Model file for the job. Use its own axes, mm. A direction names the side the tool comes from. Coordinates: 2 decimals unless noted, no trailing zeros. Write each loop counter-clockwise with the first axis right and the second up, starting at its lowest first coordinate (ties: lowest second). Pieces come first, ordered by that corner, then holes. Notation, with made-up numbers: (3.25, 58.25) - (58.25, 58.25) arc R13 ccw to (58.25, 70.25) - close; hole circle Ø8 at (-22, 52). An arc over 180 degrees is marked (long way). Put each result on its own line as item: value. Start each with the question number.
1. Pull direction Y, two halves, no side cores. Call faces 1 (the face through (10.19, 15, 99)), 2 (the face through (18.717, -18.647, 98.6)), 3 (the face through (-17, -2.966, 99)), 4 (the face through (5.385, 17, 99)): released by +Y, released by -Y, zero draft, split by the parting line, or undercut.
2. Which spindle directions (+Z, -Z, +X, -X, +Y, -Y) get a long thin tool onto all of the face, cutting with end or side? Do faces 5 (the face through (-11, -20, 99)), 6 (the face through (18.2, -8, 99)), 7 (the face through (17, 2.966, 99)). Say none if no direction does.
3. Saw through at A-A, the plane y = -8. Write the cut outline in (x, z), plus the area to 3 significant figures.
4. Saw through at B-B, the plane z = 111.5. Give the number of separate pieces and of enclosed holes in the cut face, plus the area to 3 significant figures.
5. Drill centre lines: L1, parallel to Y at x = 16, z = 160; L2, parallel to Y at x = -14, z = 22. Where is each one in solid material? Low to high. Write a range as from..to.
6. Drop flat-ended pins along their axis: P1, Ø2, axis at x = -3, y = 8, coming from the -Z side; P2, Ø2, axis at x = 17.5, z = 91, coming from the -Y side; P3, Ø0.8, axis at x = -19.5, z = 74, coming from the +Y side; P4, Ø1, axis at y = 1.5, z = 123.5, coming from the +X side. Give the stop position or say it passes through.
```python
from build123d import *

# Parameters (mm, degrees)
BOSS_EXTRUDE1_DEPTH  = 200
MIRROR3_COPY_1_DEPTH = 200
MIRROR3_COPY_2_DEPTH = 200


with BuildPart() as part:
    # Sketch1 → Boss-Extrude1 (new body)
    with BuildSketch(Plane.XY):
        with BuildLine():
            Line((3.4, 0), (5.5, 0))
            Line((5.5, 0), (5.5, 4))
            Line((5.5, 4), (11.69, 10.19))
            Line((11.69, 10.19), (18.2, 10.19))
            Line((18.2, 10.19), (18.2, 5.265595036))
            Line((18.2, 5.265595036), (15.5, 5.265595036))
            Line((15.5, 5.265595036), (15.5, 2.965595036))
            Line((15.5, 2.965595036), (19, 2.965595036))
            Line((19, 2.965595036), (19, 3.965595036))
            Line((19, 3.965595036), (20, 3.965595036))
            Line((20, 3.965595036), (20, 15.5))
            ThreePointArc((20, 15.5), (18.681980515, 18.681980515), (15.5, 20))
            Line((15.5, 20), (6.385304712, 20))
            Line((6.385304712, 20), (6.385304712, 19))
            Line((6.385304712, 19), (5.385304712, 19))
            Line((5.385304712, 19), (5.385304712, 15.5))
            Line((5.385304712, 15.5), (7.685304712, 15.5))
            Line((7.685304712, 15.5), (7.685304712, 18.2))
            Line((7.685304712, 18.2), (10.19, 18.2))
            Line((10.19, 18.2), (10.19, 11.69))
            Line((10.19, 11.69), (4, 5.5))
            Line((4, 5.5), (0, 5.5))
            Line((0, 5.5), (0, 3.4))
            ThreePointArc((0, 3.4), (2.404163056, 2.404163056), (3.4, 0))
        make_face()
        with BuildLine():
            Line((18.5, 11.69), (18.5, 15.5))
            ThreePointArc((18.5, 15.5), (17.621320344, 17.621320344), (15.5, 18.5))
            Line((15.5, 18.5), (11.69, 18.5))
            Line((11.69, 18.5), (11.69, 11.69))
            Line((11.69, 11.69), (18.5, 11.69))
        make_face(mode=Mode.SUBTRACT)
    boss_extrude1 = extrude(amount=BOSS_EXTRUDE1_DEPTH)

    # Mirror1: Boss-Extrude1 across plane
    add(boss_extrude1.mirror(Plane.ZX))

    # Mirror2: Boss-Extrude1 across plane
    add(boss_extrude1.mirror(Plane(origin=(0, 0, 0), x_dir=(0, 0, 1), z_dir=(1, 0, 0))))

    # Mirror3 copy 1 sketch → Mirror3 copy 1 (add)
    with BuildSketch(Plane(origin=(0, 0, 0), x_dir=(-1, 0, 0), z_dir=(0, 0, 1))):
        with BuildLine():
            Line((3.4, 0), (5.5, 0))
            Line((5.5, 0), (5.5, 4))
            Line((5.5, 4), (11.69, 10.19))
            Line((11.69, 10.19), (18.2, 10.19))
            Line((18.2, 10.19), (18.2, 5.265595036))
            Line((18.2, 5.265595036), (15.5, 5.265595036))
            Line((15.5, 5.265595036), (15.5, 2.965595036))
            Line((15.5, 2.965595036), (19, 2.965595036))
            Line((19, 2.965595036), (19, 3.965595036))
            Line((19, 3.965595036), (20, 3.965595036))
            Line((20, 3.965595036), (20, 15.5))
            ThreePointArc((20, 15.5), (18.681980515, 18.681980515), (15.5, 20))
            Line((15.5, 20), (6.385304712, 20))
            Line((6.385304712, 20), (6.385304712, 19))
            Line((6.385304712, 19), (5.385304712, 19))
            Line((5.385304712, 19), (5.385304712, 15.5))
            Line((5.385304712, 15.5), (7.685304712, 15.5))
            Line((7.685304712, 15.5), (7.685304712, 18.2))
            Line((7.685304712, 18.2), (10.19, 18.2))
            Line((10.19, 18.2), (10.19, 11.69))
            Line((10.19, 11.69), (4, 5.5))
            Line((4, 5.5), (0, 5.5))
            Line((0, 5.5), (0, 3.4))
            ThreePointArc((0, 3.4), (2.404163056, 2.404163056), (3.4, 0))
        make_face()
        with BuildLine():
            Line((18.5, 11.69), (18.5, 15.5))
            ThreePointArc((18.5, 15.5), (17.621320344, 17.621320344), (15.5, 18.5))
            Line((15.5, 18.5), (11.69, 18.5))
            Line((11.69, 18.5), (11.69, 11.69))
            Line((11.69, 11.69), (18.5, 11.69))
        make_face(mode=Mode.SUBTRACT)
    extrude(amount=MIRROR3_COPY_1_DEPTH)

    # Mirror3 copy 2 sketch → Mirror3 copy 2 (add)
    with BuildSketch(Plane.XY):
        with BuildLine():
            Line((3.4, 0), (5.5, 0))
            Line((5.5, 0), (5.5, -4))
            Line((5.5, -4), (11.69, -10.19))
            Line((11.69, -10.19), (18.2, -10.19))
            Line((18.2, -10.19), (18.2, -5.265595036))
            Line((18.2, -5.265595036), (15.5, -5.265595036))
            Line((15.5, -5.265595036), (15.5, -2.965595036))
            Line((15.5, -2.965595036), (19, -2.965595036))
            Line((19, -2.965595036), (19, -3.965595036))
            Line((19, -3.965595036), (20, -3.965595036))
            Line((20, -3.965595036), (20, -15.5))
            ThreePointArc((20, -15.5), (18.681980515, -18.681980515), (15.5, -20))
            Line((15.5, -20), (6.385304712, -20))
            Line((6.385304712, -20), (6.385304712, -19))
            Line((6.385304712, -19), (5.385304712, -19))
            Line((5.385304712, -19), (5.385304712, -15.5))
            Line((5.385304712, -15.5), (7.685304712, -15.5))
            Line((7.685304712, -15.5), (7.685304712, -18.2))
            Line((7.685304712, -18.2), (10.19, -18.2))
            Line((10.19, -18.2), (10.19, -11.69))
            Line((10.19, -11.69), (4, -5.5))
            Line((4, -5.5), (0, -5.5))
            Line((0, -5.5), (0, -3.4))
            ThreePointArc((0, -3.4), (2.404163056, -2.404163056), (3.4, 0))
        make_face()
        with BuildLine():
            Line((18.5, -11.69), (18.5, -15.5))
            ThreePointArc((18.5, -15.5), (17.621320344, -17.621320344), (15.5, -18.5))
            Line((15.5, -18.5), (11.69, -18.5))
            Line((11.69, -18.5), (11.69, -11.69))
            Line((11.69, -11.69), (18.5, -11.69))
        make_face(mode=Mode.SUBTRACT)
    extrude(amount=MIRROR3_COPY_2_DEPTH)


solid = part.part
```
Final values:
1. face 1: undercut
1. face 2: released by -Y
1. face 3: undercut
1. face 4: zero draft
2. face 5: +Z, -Z, +X, -X, -Y
2. face 6: +Z, -Z
2. face 7: +Z, -Z, +X
3. outline: (-20, 0) - (-18.2, 0) - (-18.2, 200) - (-20, 200) - close; (-9.5, 0) - (-6.5, 0) - (-6.5, 200) - (-9.5, 200) - close; (6.5, 0) - (9.5, 0) - (9.5, 200) - (6.5, 200) - close; (18.2, 0) - (20, 0) - (20, 200) - (18.2, 200) - close
3. area: 1,920 mm²
4. separate pieces: 1
4. enclosed holes: 5
4. area: 468 mm²
5. L1: y = -19.97..-18.46, -11.69..-10.19, -5.27..-2.97, 2.97..5.27, 10.19..11.69, 18.46..19.97
5. L2: y = -20..-18.5, -11.69..-10.19, 10.19..11.69, 18.5..20
6. P1: passes through
6. P2: stops at y = -19.89
6. P3: stops at y = 18.2
6. P4: stops at x = 5.5
